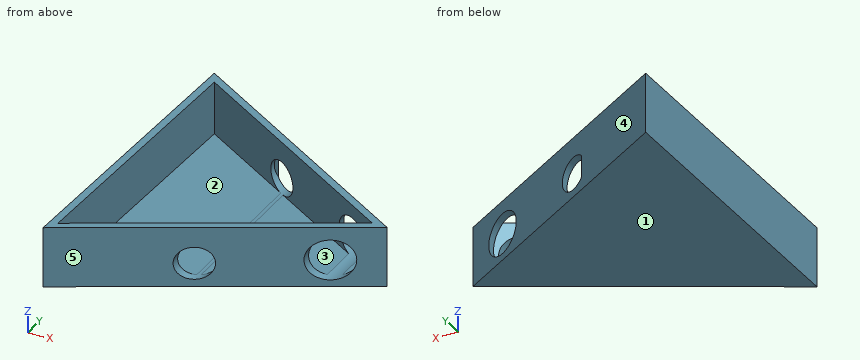
from build123d import *

# Parameters (mm, degrees)
F1_DEPTH = 8
F2_T     = -1
F3_R     = 2.170794
F3_R_2   = 2.696969
F4_DEPTH = 12.5


with BuildPart() as f1:
    # F0 (on Top) → F1 (new body)
    with BuildSketch(Plane.XY):
        Polygon((-12.137679, -19.559744), (23.008074, -0.731667), (-10.870395, 20.29141), align=None)
    extrude(amount=F1_DEPTH)

    # F2
    f2_openings = [f1.faces().sort_by_distance(p)[0] for p in [
        (0, 0, 8),
    ]]
    offset(amount=F2_T, openings=f2_openings)

    # F3 (on Front) → F4 (cut, symmetric)
    with BuildSketch(Plane.XZ):
        with Locations((3.323053, 3.15884)):
            Circle(F3_R)
        with Locations((17.222516, 3.580036)):
            Circle(F3_R_2)
    extrude(amount=F4_DEPTH, both=True, mode=Mode.SUBTRACT)


solid = f1.part
The model under review builds one solid part; all positions refer to its coordinate system, in mm. Face numbers are marked on the shaded views. A direction names the side the tool comes from. Round coordinates to 2 decimals unless told otherwise and drop trailing zeros. Order: outer loops, then holes, each group sorted by start corner. A loop starts at its lowest first (then second) coordinate and runs counter-clockwise, first axis right, second up. Notation, with made-up numbers: (33, -27) -> (87, -27) arc R21 ccw to (87, -7) -> close; hole circle Ø4 at (-11.5, -18.5). An arc over 180 degrees is marked (long way). Write item = value, one per line. Start each with the question number.
Item 1: For line 1 along Z through (x, y) = (-9.5, 4); line 2 along Y through (x, z) = (20.5, 2); line 3 along X through (y, z) = (15, 3.25), list the stretches that pass through material, from the lowest coordinate up.
Item 2: Consider section B-B on z = 7. Write out the cut boundary in (x, y).
Item 3: Mouldability with a two-part tool opening along Y and no side actions: class the marked faces 3, 4 and 5 as released by +Y, released by -Y, zero draft, split by the parting line, or undercut.
Item 4: Consider section A-A on y = -4. Write out the cut boundary in (x, z).
Item 5: For the marked faces 1 and 2, list the 3-axis set-ups (+Z, -Z, +X, -X, +Y, -Y) from which the entire face can be reached by the end or side of a thin tool; tool diameter is ignored.
Item 6: Consider section C-C on x = 5. Write out the cut boundary in (y, z).
Item 7: Consider section D-D on y = -16. Write out the cut boundary in (x, z), plus the area to 3 significant figures.
Item 8: Clearance check with flat-ended pins moving along their axes: pin 1 Ø3 at (x, z) = (-4.5, 6) entering from +Y; pin 2 Ø1 at (x, z) = (12.5, 5.5) entering from -Y; pin 3 Ø3.5 at (x, y) = (19, -1) entering from +Z; pin 4 Ø7 at (x, y) = (-2, -8) entering from +Z. State where each tip first meets the part, or that it passes through.
Conclusion:
q1.line_1 = 0 to 1
q1.line_2 = -2.08 to -0.94, -0.35 to 0.82
q1.line_3 = -11.04 to -10.04, -4.24 to -2.34
q2.outline = (-12.14, -19.56) -> (23.01, -0.73) -> (-10.87, 20.29) -> close; hole (-11.08, -17.86) -> (21.01, -0.67) -> (-9.93, 18.53) -> close
q3.face_3 = undercut
q3.face_4 = released by +Y
q3.face_5 = released by -Y
q4.outline = (-11.64, 0) -> (16.91, 0) -> (16.91, 0.9) arc R2.7 cw to (14.79, 2.42) -> (14.79, 1) -> (3.55, 1) arc R2.17 cw to (3.1, 1) -> (-10.64, 1) -> (-10.64, 8) -> (-11.64, 8) -> close; (14.79, 4.74) arc R2.7 cw to (16.91, 6.26) -> (16.91, 8) -> (14.79, 8) -> close
q5.face_1 = -Z, +X, -X, +Y, -Y
q5.face_2 = +Z
q6.outline = (-10.38, 0) -> (10.44, 0) -> (10.44, 1.78) -> (9.27, 1.78) -> (9.27, 1) -> (-9.24, 1) -> (-9.24, 1.78) -> (-10.38, 1.78) -> close; (-10.38, 4.54) -> (-9.24, 4.54) -> (-9.24, 8) -> (-10.38, 8) -> close; (9.27, 4.54) -> (10.44, 4.54) -> (10.44, 8) -> (9.27, 8) -> close
q7.outline = (-12.02, 0) -> (-5.49, 0) -> (-5.49, 8) -> (-7.61, 8) -> (-7.61, 1) -> (-11.02, 1) -> (-11.02, 8) -> (-12.02, 8) -> close
q7.area = 28.4 mm2
q8.pin_1 = 17.27
q8.pin_2 = -6.63
q8.pin_3 = 8
q8.pin_4 = 1
